Check sheet for the drawn part. Datum: minimum x, y, z corner. Units: mm. A direction names the side the tool comes from. Coordinates: 2 decimals unless noted, no trailing zeros. Loops run counter-clockwise (first coordinate to the right, second up) from the corner with the lowest first, then second, coordinate; pieces in that order, holes last.
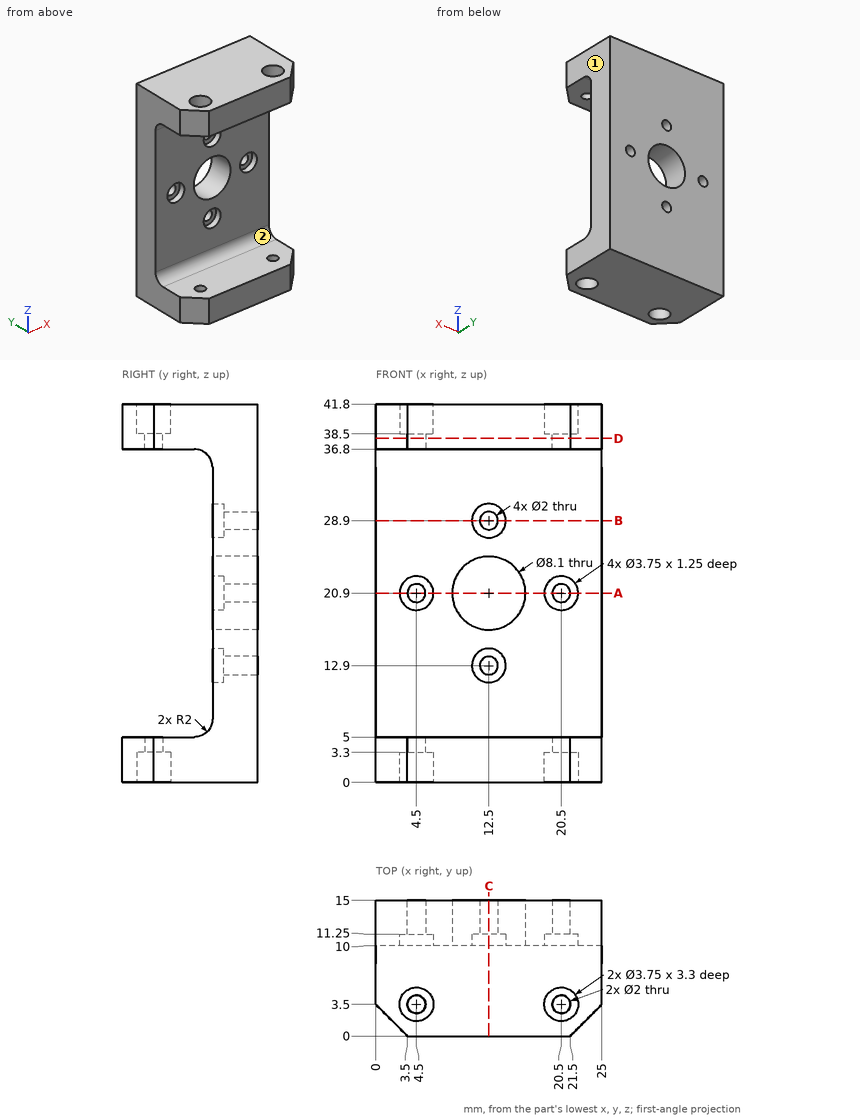
1) Section check C-C on x = 12.5. Give the number of separate pieces and of enclosed holes in the cut face, plus the area to 3 significant figures.
Answer sheet:
separate pieces: 4
enclosed holes: 0
area: 246 mm2
2) Section check D-D on z = 38. Enter the section's corners in (x, y), plus the area to 3 significant figures.
Answer sheet:
outline: (0, 3.5) - (3.5, 0) - (21.5, 0) - (25, 3.5) - (25, 15) - (0, 15) - close; hole circle Ø2 at (4.5, 3.5); hole circle Ø2 at (20.5, 3.5)
area: 356 mm2
3) Set-up check for the marked faces 1 and 2: record each of +Z, -Z, +X, -X, +Y, -Y from which the full face is reachable in a straight line by a thin tool's end or side.
Answer sheet:
face 1: +Z, -Z, +X, +Y, -Y
face 2: +X, -X, -Y
4) Section check B-B on z = 28.9. Enter the section's corners in (x, y) (3 decimals).
Answer sheet:
outline: (0, 10) - (10.625, 10) - (10.625, 11.25) - (11.5, 11.25) - (11.5, 15) - (0, 15) - close; (13.5, 11.25) - (14.375, 11.25) - (14.375, 10) - (25, 10) - (25, 15) - (13.5, 15) - close
5) Scan lines: line 1 (Z direction, x = 4.5, y = 10.95) (3 decimals); line 2 (Z direction, x = 21.25, y = 1.5); line 3 (Y direction, x = 4.5, z = 39.5) (3 decimals). Record each from-to range of solid material in increasing order.
Answer sheet:
line 1: z = 0 to 19.025, 22.775 to 41.8
line 2: z = 0 to 5, 36.8 to 41.8
line 3: y = 0 to 1.625, 5.375 to 15
6) Section check A-A on z = 20.9. Enter the section's corners in (x, y) (3 decimals).
Answer sheet:
outline: (0, 10) - (2.625, 10) - (2.625, 11.25) - (3.5, 11.25) - (3.5, 15) - (0, 15) - close; (5.5, 11.25) - (6.375, 11.25) - (6.375, 10) - (8.45, 10) - (8.45, 15) - (5.5, 15) - close; (16.55, 10) - (18.625, 10) - (18.625, 11.25) - (19.5, 11.25) - (19.5, 15) - (16.55, 15) - close; (21.5, 11.25) - (22.375, 11.25) - (22.375, 10) - (25, 10) - (25, 15) - (21.5, 15) - close
7) Depth check by flat-ended pin: pin 1 (12 mm diameter, centred on x = 12, z = 26.5, fed in from -Y); pin 2 (3 mm diameter, centred on x = 20.5, y = 3.5, fed in from -Z); pin 3 (5 mm diameter, centred on y = 5.5, z = 24, fed in from -X); pin 4 (1.9 mm diameter, centred on x = 20.5, y = 3, fed in from +Z). Enter the tip coordinate at first touch or a pass-through.
Answer sheet:
pin 1: stops at y = 10
pin 2: stops at z = 3.3
pin 3: passes through
pin 4: stops at z = 38.5
